from build123d import *

# Parameters (mm, degrees)
SKETCH1_R             = 4.7625
BOSS_EXTRUDE1_DEPTH   = 50.8
BOSS_EXTRUDE1_2_DEPTH = 50.8
BOSS_EXTRUDE1_3_DEPTH = 50.8
BOSS_EXTRUDE1_4_DEPTH = 50.8
SKETCH2_W             = 67.765000106
SKETCH2_H             = 90.2184886
BOSS_EXTRUDE2_DEPTH   = 12.7
CUT_EXTRUDE1_START    = -0.7366
F_3DSKETCH1_R         = 4.7625
CUT_EXTRUDE1_DEPTH    = 0.7366
SKETCH3_R             = 4.4704
BOSS_EXTRUDE3_DEPTH   = 0.7366
F_3DSKETCH2_R         = 5.08
CUT_EXTRUDE2_DEPTH    = 0.7366
SKETCH4_R             = 4.4704
BOSS_EXTRUDE4_DEPTH   = 0.7366


with BuildPart() as part:
    # Sketch1 → Boss-Extrude1 (new body)
    with BuildSketch(Plane(origin=(0, 0, 0), x_dir=(1, 0, 0), z_dir=(0, 1, 0))):
        with Locations(Location((-29.1199951, 40.3467443, 0), (0, 0, 270))):
            Circle(SKETCH1_R)
    extrude(amount=BOSS_EXTRUDE1_DEPTH)



with BuildPart() as body_2:
    # Sketch1 → Boss-Extrude1 2 (new body)
    with BuildSketch(Plane(origin=(0, 0, 0), x_dir=(1, 0, 0), z_dir=(0, 1, 0))):
        with Locations(Location((-29.1199951, -40.3467443, 0), (0, 0, 270))):
            Circle(SKETCH1_R)
    extrude(amount=BOSS_EXTRUDE1_2_DEPTH)


with BuildPart() as body_3:
    # Sketch1 → Boss-Extrude1 3 (new body)
    with BuildSketch(Plane(origin=(0, 0, 0), x_dir=(1, 0, 0), z_dir=(0, 1, 0))):
        with Locations(Location((29.120005006, -40.3467443, 0), (0, 0, 270))):
            Circle(SKETCH1_R)
    extrude(amount=BOSS_EXTRUDE1_3_DEPTH)


with BuildPart() as body_4:
    # Sketch1 → Boss-Extrude1 4 (new body)
    with BuildSketch(Plane(origin=(0, 0, 0), x_dir=(1, 0, 0), z_dir=(0, 1, 0))):
        with Locations(Location((29.120005006, 40.3467443, 0), (0, 0, 270))):
            Circle(SKETCH1_R)
    extrude(amount=BOSS_EXTRUDE1_4_DEPTH)


with BuildPart() as part_1:
    add(part.part)

    add(body_2.part)  # Boss-Extrude2 merges body 2

    add(body_3.part)  # Boss-Extrude2 merges body 3

    add(body_4.part)  # Boss-Extrude2 merges body 4
    # Sketch2 → Boss-Extrude2 (add)
    with BuildSketch(Plane(origin=(0, 50.8, 0), x_dir=(1, 0, 0), z_dir=(0, 1, 0))):
        with Locations((4.953e-06, 0)):
            Rectangle(SKETCH2_W, SKETCH2_H)
    extrude(amount=BOSS_EXTRUDE2_DEPTH)

    # 3DSketch1 → Cut-Extrude1 (cut)
    with BuildSketch(Plane(origin=(-29.1199951, 12.7, 40.3467443), x_dir=(0.5852354085547554, 0, -0.8108634389178911), z_dir=(0, 1, 0)).offset(CUT_EXTRUDE1_START)):
        with Locations(Location((0, 0, 0), (0, 0, 35.819622287))):
            Circle(F_3DSKETCH1_R)
        with Locations(Location((34.084110256, -47.224686769, 0), (0, 0, 35.819622287))):
            Circle(F_3DSKETCH1_R)
        with Locations(Location((99.515509921, 0, 0), (0, 0, 35.819622287))):
            Circle(F_3DSKETCH1_R)
        with Locations(Location((65.431399664, 47.224686769, 0), (0, 0, 35.819622287))):
            Circle(F_3DSKETCH1_R)
    extrude(amount=CUT_EXTRUDE1_DEPTH, mode=Mode.SUBTRACT)


with BuildPart() as cut_extrude1_piece_1:
    # of the separate pieces the step leaves, piece 1, a body of its own (cut_extrude1_pieces)
    add(part_1.part.solids().sort_by_distance((-29.1199951, 12.7, -35.5842443))[0])



with BuildPart() as cut_extrude1_piece_2:
    # of the separate pieces the step leaves, piece 2, a body of its own (cut_extrude1_pieces)
    add(part_1.part.solids().sort_by_distance((-29.1199951, 0, 45.1092443))[0])


with BuildPart() as cut_extrude1_piece_3:
    # of the separate pieces the step leaves, piece 3, a body of its own (cut_extrude1_pieces)
    add(part_1.part.solids().sort_by_distance((-29.1199951, 0, -35.5842443))[0])


with BuildPart() as cut_extrude1_piece_4:
    # of the separate pieces the step leaves, piece 4, a body of its own (cut_extrude1_pieces)
    add(part_1.part.solids().sort_by_distance((29.120005006, 0, -35.5842443))[0])


with BuildPart() as cut_extrude1_piece_5:
    # of the separate pieces the step leaves, piece 5, a body of its own (cut_extrude1_pieces)
    add(part_1.part.solids().sort_by_distance((29.120005006, 0, 45.1092443))[0])


with BuildPart() as cut_extrude1_piece_1_1:
    add(cut_extrude1_piece_1.part)

    add(cut_extrude1_piece_2.part)  # Boss-Extrude3 merges Cut-Extrude1 piece 2

    add(cut_extrude1_piece_3.part)  # Boss-Extrude3 merges Cut-Extrude1 piece 3

    add(cut_extrude1_piece_4.part)  # Boss-Extrude3 merges Cut-Extrude1 piece 4

    add(cut_extrude1_piece_5.part)  # Boss-Extrude3 merges Cut-Extrude1 piece 5
    # Sketch3 → Boss-Extrude3 (add)
    with BuildSketch(Plane(origin=(0, 12.7, 0), x_dir=(-1, 0, 0), z_dir=(0, -1, 0))):
        with Locations(Location((29.1199951, 40.3467443, 0), (0, 0, 90))):
            Circle(SKETCH3_R)
        with Locations(Location((-29.120005006, 40.3467443, 0), (0, 0, 90))):
            Circle(SKETCH3_R)
        with Locations(Location((-29.120005006, -40.3467443, 0), (0, 0, 90))):
            Circle(SKETCH3_R)
        with Locations(Location((29.1199951, -40.3467443, 0), (0, 0, 90))):
            Circle(SKETCH3_R)
    extrude(amount=BOSS_EXTRUDE3_DEPTH)

    # 3DSketch2 → Cut-Extrude2 (cut)
    with BuildSketch(Plane(origin=(-29.1199951, 19.05, 40.3467443), x_dir=(0.5852354085547554, 0, -0.8108634389178911), z_dir=(0, 1, 0))):
        Circle(F_3DSKETCH2_R)
        with Locations((34.084110256, -47.224686769)):
            Circle(F_3DSKETCH2_R)
        with Locations((99.515509921, 0)):
            Circle(F_3DSKETCH2_R)
        with Locations((65.431399664, 47.224686769)):
            Circle(F_3DSKETCH2_R)
    extrude(amount=CUT_EXTRUDE2_DEPTH, mode=Mode.SUBTRACT)


with BuildPart() as cut_extrude2_piece_1:
    # of the separate pieces the step leaves, piece 1, a body of its own (cut_extrude2_pieces)
    add(cut_extrude1_piece_1_1.part.solids().sort_by_distance((29.120005006, 19.7866, 45.1092443))[0])



with BuildPart() as cut_extrude2_piece_2:
    # of the separate pieces the step leaves, piece 2, a body of its own (cut_extrude2_pieces)
    add(cut_extrude1_piece_1_1.part.solids().sort_by_distance((-29.1199951, 12.7, 45.1092443))[0])


with BuildPart() as cut_extrude2_piece_3:
    # of the separate pieces the step leaves, piece 3, a body of its own (cut_extrude2_pieces)
    add(cut_extrude1_piece_1_1.part.solids().sort_by_distance((-29.1199951, 12.7, -35.5842443))[0])


with BuildPart() as cut_extrude2_piece_4:
    # of the separate pieces the step leaves, piece 4, a body of its own (cut_extrude2_pieces)
    add(cut_extrude1_piece_1_1.part.solids().sort_by_distance((29.120005006, 12.7, -35.5842443))[0])


with BuildPart() as cut_extrude2_piece_5:
    # of the separate pieces the step leaves, piece 5, a body of its own (cut_extrude2_pieces)
    add(cut_extrude1_piece_1_1.part.solids().sort_by_distance((29.120005006, 0, 45.1092443))[0])


with BuildPart() as cut_extrude2_piece_1_1:
    add(cut_extrude2_piece_1.part)

    add(cut_extrude2_piece_2.part)  # Boss-Extrude4 merges Cut-Extrude2 piece 2

    add(cut_extrude2_piece_3.part)  # Boss-Extrude4 merges Cut-Extrude2 piece 3

    add(cut_extrude2_piece_4.part)  # Boss-Extrude4 merges Cut-Extrude2 piece 4

    add(cut_extrude2_piece_5.part)  # Boss-Extrude4 merges Cut-Extrude2 piece 5
    # Sketch4 → Boss-Extrude4 (add)
    with BuildSketch(Plane(origin=(0, 19.7866, 0), x_dir=(-1, 0, 0), z_dir=(0, -1, 0))):
        with Locations(Location((29.1199951, -40.3467443, 0), (0, 0, 270))):
            Circle(SKETCH4_R)
        with Locations(Location((-29.120005006, -40.3467443, 0), (0, 0, 270))):
            Circle(SKETCH4_R)
        with Locations(Location((-29.120005006, 40.3467443, 0), (0, 0, 270))):
            Circle(SKETCH4_R)
        with Locations(Location((29.1199951, 40.3467443, 0), (0, 0, 270))):
            Circle(SKETCH4_R)
    extrude(amount=BOSS_EXTRUDE4_DEPTH)


solid = cut_extrude2_piece_1_1.part
CAD build for the part. Positions are in the model's coordinates, mm. A direction names the side the tool comes from. Give positions to 0.01 mm unless a question says otherwise; leave off trailing zeros. Loops run counter-clockwise (first coordinate to the right, second up) from the corner with the lowest first, then second, coordinate; pieces in that order, holes last. Notation, with made-up numbers: M 56.5,83 L 86.5,83 A20 cw 86.5,122 Z; hole C -6,33.25 d7. An arc over 180 degrees is marked long. One line per question, with ' | ' between items. Start each with the question number.
1. Probe L1, parallel to Y at x = 7.5, z = 13; L2, parallel to X at y = 24.5, z = 38.5; L3, parallel to X at y = 10, z = -37. List the from-to ranges inside material, lowest first. Write a range as from..to.
2. 3-axis set-ups, long thin cutter, end or side, ignore diameter. For faces 1 (the face through (-33.883, 57, 1)), 2 (the face through (-30.944, 15.831, 44.746)), 3 (the face through (-29, 0, 40)), 4 (the face through (-25.154, 19.423, 42.41)), 5 (the face through (33, 50.8, -44)): which of +Z, -Z, +X, -X, +Y, -Y reach the whole face in a straight line?
3. Flat gauge pins, fed straight in: pin 1 (3 mm diameter, centred on x = 24, z = -5.5, fed in from -Y); pin 2 (1.5 mm diameter, centred on x = 24.5, y = 25.5, fed in from +Z). Where does each tip first touch, or does it go through?
4. Saw through at C-C on x = 7.5. Give the cut face in (y, z).
5. Saw through at B-B on z = 21.5. Give the cut face in (x, y), plus the area to 3 significant figures.
6. Saw through at A-A on y = 42. Give the cut face in (x, z) (1 decimal).
7. Two-plate mould, pull along Y, no slides. Class faces 6 (the face through (-25.1, 35.1, 42.9)), 7 (the face through (29, 0, 40)), 8 (the face through (-24.69, 12.34, -39.76)): pulls with the +Y half, pulls with the -Y half, needs draft (parallel to the pull), parting line crosses it, or undercut.
Result sheet:
1) L1: y = 50.8..63.5 | L2: x = -33.51..-24.73, 24.73..33.51 | L3: x = -32.51..-25.73, 25.73..32.51
2) face 1: +Z, -Z, -X, +Y, -Y | face 2: -Y | face 3: +Z, -Z, +X, -X, -Y | face 4: none | face 5: -Z, +X, -Y
3) pin 1: stops at y = 50.8 | pin 2: stops at z = 43.12
4) outline: M 50.8,-45.11 L 63.5,-45.11 L 63.5,45.11 L 50.8,45.11 Z
5) outline: M -33.88,50.8 L 33.88,50.8 L 33.88,63.5 L -33.88,63.5 Z | area: 861 mm^2
6) outline: C -29.1,-40.3 d9.5; C -29.1,40.3 d9.5; C 29.1,-40.3 d9.5; C 29.1,40.3 d9.5
7) face 6: needs draft | face 7: pulls with the -Y half | face 8: undercut
